Part model, mm, in its own coordinate system. Face numbers are marked on the shaded views. A direction names the side the tool comes from. Coordinates: 2 decimals unless noted, no trailing zeros. Loops run counter-clockwise (first coordinate to the right, second up) from the corner with the lowest first, then second, coordinate; pieces in that order, holes last. Notation, with made-up numbers: (13, -9.75) -> (49, -9.75) arc R19 cw to (49, 8.25) -> close; hole circle Ø7 at (-9.5, -37.75). An arc over 180 degrees is marked (long way). Use one line per item in the form item = value. Start each with the question number.
(1) Band-saw the part on A-A on x = 6. Give the cut face in (y, z).
(2) Mould opens along Y. For the marked faces 1, 2, 3 and 4 say: +Y half, -Y half, draft (parallel to the pull), parting line (faces both ways), or undercut.
(3) Band-saw the part on C-C on x = 12. Give the cut face in (y, z), then the cut area to 3 significant figures.
(4) Pin check, flat tips, straight feed: P1, Ø6.5, axis at x = -12, y = 0.5, coming from the -Z side; P2, Ø11, axis at y = -18.5, z = 4, coming from the +X side; P3, Ø4, axis at x = 14, y = -37.5, coming from the -Z side. Stop position of each tip, or through.
(5) 3-axis set-ups, long thin cutter, end or side, ignore diameter. For the marked faces 5, 6, 7, 8 and 9: which of +Z, -Z, +X, -X, +Y, -Y reach the whole face in a straight line?
(6) Band-saw the part on B-B on y = -28. Give the cut face in (x, z).
(7) Band-saw the part on D-D on x = 0. Give the cut face in (y, z), then the cut area to 3 significant figures.
(8) Drill centre lines: L1, parallel to Y at x = 13, z = 5.9; L2, parallel to Y at x = -13, z = 1.15; L3, parallel to X at y = -38, z = 2.1. Where is each one in solid material? Low to high. Write a range as [from, to].
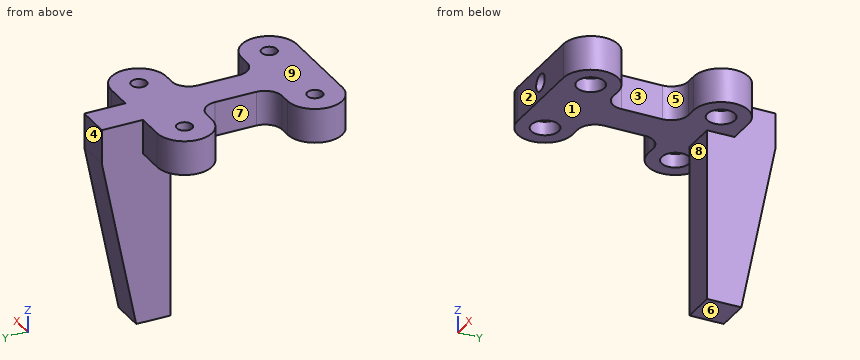
```python
from build123d import *

# Parameters (mm, degrees)
F0_R     = 2.25
F1_DEPTH = 10
F2_W     = 12
F2_H     = 10
F3_DEPTH = 10
F4_R     = 2.45
F5_DEPTH = 25
F6_R     = 4
F7_DEPTH = 4


with BuildPart() as f1:
    # F0 (on Top) → F1 (new body)
    with BuildSketch(Plane.XY):
        with BuildLine():
            Line((13, 8), (0, 8))
            Line((0, 8), (-13, 8))
            ThreePointArc((-13, 8), (-21, 0), (-13, -8))
            Line((-13, -8), (-10, -8))
            ThreePointArc((-10, -8), (-6.464466, -9.464466), (-5, -13))
            Line((-5, -13), (-5, -25))
            ThreePointArc((-5, -25), (-6.464466, -28.535534), (-10, -30))
            Line((-10, -30), (-13, -30))
            ThreePointArc((-13, -30), (-21, -38), (-13, -46))
            Line((-13, -46), (0, -46))
            Line((0, -46), (13, -46))
            ThreePointArc((13, -46), (21, -38), (13, -30))
            Line((13, -30), (10, -30))
            ThreePointArc((10, -30), (6.464466, -28.535534), (5, -25))
            Line((5, -25), (5, -13))
            ThreePointArc((5, -13), (6.464466, -9.464466), (10, -8))
            Line((10, -8), (13, -8))
            ThreePointArc((13, -8), (21, 0), (13, 8))
        make_face()
        with Locations((-13, -38)):
            Circle(F0_R, mode=Mode.SUBTRACT)
        with Locations((13, -38)):
            Circle(F0_R, mode=Mode.SUBTRACT)
        with Locations((-13, 0)):
            Circle(F0_R, mode=Mode.SUBTRACT)
        with Locations((13, 0)):
            Circle(F0_R, mode=Mode.SUBTRACT)
    extrude(amount=F1_DEPTH)

    # F2 (on face) → F3 (join)
    with BuildSketch(Plane.YZ.offset(5)):
        Polygon((8, 0), (0, 0), (0, -50), (10, -50), (20, 0), align=None)
        with Locations((14, 5)):
            Rectangle(F2_W, F2_H)
    extrude(amount=-F3_DEPTH)

    # F4 (on face) → F5 (cut)
    with BuildSketch(Plane.XZ.offset(46)):
        with Locations((0, 5)):
            Circle(F4_R)
    extrude(amount=-F5_DEPTH, mode=Mode.SUBTRACT)

    # F6 (on face) → F7 (cut)
    with BuildSketch(Plane(origin=(0, 0, 0), x_dir=(1, 0, 0), z_dir=(0, 0, -1))):
        with Locations((13, 0)):
            Circle(F6_R)
        with Locations((-13, 0)):
            Circle(F6_R)
        with Locations((-13, 38)):
            Circle(F6_R)
        with Locations((13, 38)):
            Circle(F6_R)
    extrude(amount=-F7_DEPTH, mode=Mode.SUBTRACT)


solid = f1.part
```
A:
q1.outline = (-46, 0) -> (-28, 0) -> (-28, 10) -> (-46, 10) -> close; (-10, 0) -> (8, 0) -> (8, 10) -> (-10, 10) -> close
q2.face_1 = draft
q2.face_2 = -Y half
q2.face_3 = undercut
q2.face_4 = +Y half
q3.outline = (-46, 0) -> (-41.87, 0) -> (-41.87, 4) -> (-40.02, 4) -> (-40.02, 10) -> (-46, 10) -> close; (-35.98, 4) -> (-34.13, 4) -> (-34.13, 0) -> (-30, 0) -> (-30, 10) -> (-35.98, 10) -> close; (-8, 0) -> (-3.87, 0) -> (-3.87, 4) -> (-2.02, 4) -> (-2.02, 10) -> (-8, 10) -> close; (2.02, 4) -> (3.87, 4) -> (3.87, 0) -> (8, 0) -> (8, 10) -> (2.02, 10) -> close
q3.area = 210 mm²
q4.P1 = 0
q4.P2 = 5
q4.P3 = 4
q5.face_5 = +Z, -Z, +X
q5.face_6 = -Z, +X, -X, +Y, -Y
q5.face_7 = +Z, -Z, -X
q5.face_8 = -Z, +X, -X, -Y
q5.face_9 = +Z, +X, -X, +Y, -Y
q6.outline = (-6, 0) -> (6, 0) -> (6, 10) -> (-6, 10) -> close; hole circle Ø4.9 at (0, 5)
q7.outline = (-46, 0) -> (0, 0) -> (0, -50) -> (10, -50) -> (20, 0) -> (20, 10) -> (-46, 10) -> (-46, 7.45) -> (-21, 7.45) -> (-21, 2.55) -> (-46, 2.55) -> close
q7.area = 1,290 mm²
q8.L1 = [-46, -40.25], [-35.75, -30], [-8, -2.25], [2.25, 8]
q8.L2 = [-46, -42], [-34, -30], [-8, -4], [4, 8]
q8.L3 = [-21, -17], [-9, 9], [17, 21]
